from build123d import *

# Parameters (mm, degrees)
SKETCH1_W               = 20
SKETCH1_H               = 20
BOSS_EXTRUDE1_DEPTH     = 3
CUT_EXTRUDE1_DEPTH      = 1
CUT_EXTRUDE1_DEPTH_BACK = 4


with BuildPart() as part:
    # Sketch1 → Boss-Extrude1 (new body)
    with BuildSketch(Plane(origin=(0, 0, 0), x_dir=(1, 0, 0), z_dir=(0, 1, 0))):
        Rectangle(SKETCH1_W, SKETCH1_H)
    extrude(amount=BOSS_EXTRUDE1_DEPTH)

    # Sketch2 → Cut-Extrude1 (cut, two sides)
    with BuildSketch(Plane(origin=(0, 3, 0), x_dir=(1, 0, 0), z_dir=(0, 1, 0))) as cut_extrude1_sk:
        Polygon((-5, -10), (-10, -5), (-10, -10), align=None)
        Polygon((0, -5), (-5, -10), (5, -10), align=None)
        Polygon((10, -5), (5, -10), (10, -10), align=None)
    extrude(amount=CUT_EXTRUDE1_DEPTH, mode=Mode.SUBTRACT)
    extrude(cut_extrude1_sk.sketch, amount=-CUT_EXTRUDE1_DEPTH_BACK, mode=Mode.SUBTRACT)


solid = part.part
Work out the finished part from the listing and answer in its coordinate system (mm). Coordinates: 2 decimals unless noted, no trailing zeros. Loops run counter-clockwise (first coordinate to the right, second up) from the corner with the lowest first, then second, coordinate; pieces in that order, holes last. Notation, with made-up numbers: (72, 65) -> (131, 65) arc R23 cw to (131, 73) -> close; hole circle Ø4 at (50, 2). An arc over 180 degrees is marked (long way). Answer as CSV lines item,"result".
1) The part is cut by section D-D (x = -4.5). Give the vertices of the cut face in (y, z), and give its area (3 significant figures).
A:
outline,"(0, -10) -> (3, -10) -> (3, 9.5) -> (0, 9.5) -> close"
area,"58.5 mm²"
2) The part is cut by section B-B (y = 1.8). Give the vertices of the cut face in (x, z).
A:
outline,"(-10, -10) -> (10, -10) -> (10, 5) -> (5, 10) -> (0, 5) -> (-5, 10) -> (-10, 5) -> close"
3) For a pull along X with two mould halves and no side action, classify faces 1 (the face through (-7, 2, 8)), 2 (the face through (3, 2, 8)), 3 (the face through (0, 0, -2)), 4 (the face through (-2, 2, 7)) as released by +X, released by -X, zero draft, split by the parting line, or undercut.
A:
face 1,"released by -X"
face 2,"undercut"
face 3,"zero draft"
face 4,"undercut"
4) Straight lines are drawn through the part: probe 1 along X at (y, z) = (2.55, 6); probe 2 along X at (y, z) = (1.7, 9); probe 3 along Z at (x, y) = (-4.25, 0.75). For each, find the intervals that lie inside material, in ascending order.
A:
probe 1,"x = -9 to -1, 1 to 9"
probe 2,"x = -6 to -4, 4 to 6"
probe 3,"z = -10 to 9.25"
5) The part is cut by section A-A (z = 8.75). Give the vertices of the cut face in (x, y), and give its area (3 significant figures).
A:
outline,"(-6.25, 0) -> (-3.75, 0) -> (-3.75, 3) -> (-6.25, 3) -> close; (3.75, 0) -> (6.25, 0) -> (6.25, 3) -> (3.75, 3) -> close"
area,"15.0 mm²"
6) The part is cut by section C-C (z = 5.75). Give the vertices of the cut face in (x, y), and give its area (3 significant figures).
A:
outline,"(-9.25, 0) -> (-0.75, 0) -> (-0.75, 3) -> (-9.25, 3) -> close; (0.75, 0) -> (9.25, 0) -> (9.25, 3) -> (0.75, 3) -> close"
area,"51.0 mm²"
